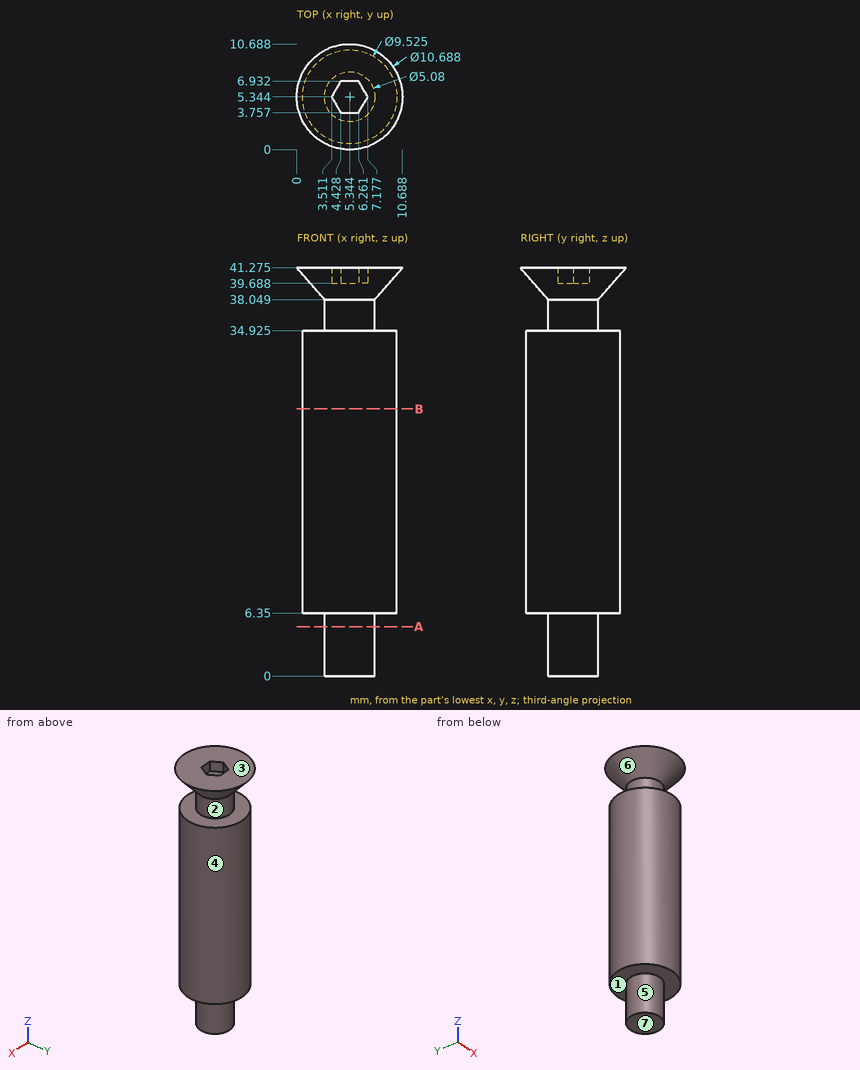
Job drawing, mm, ordinate dimensions from the low corner. One solid piece. A direction names the side the tool comes from. Give positions to 0.01 mm unless a question says otherwise; leave off trailing zeros. Write each loop counter-clockwise with the first axis right and the second up, starting at its lowest first coordinate (ties: lowest second). Pieces come first, ordered by that corner, then holes. Notation, with made-up numbers: (10, 24.5) -> (68, 24.5) arc R5 ccw to (68, 31.5) -> close; hole circle Ø1 at (-23, 39). An arc over 180 degrees is marked (long way). Return JSON: item names as keys, results as strings.
Item 1: Drop flat-ended pins along their axis: pin 1 (1.7 mm diameter, centred on x = 5.5, z = 40, fed in from +Y) (1 decimal); pin 2 (1.5 mm diameter, centred on x = 2, y = 8.5, fed in from -Z); pin 3 (0.8 mm diameter, centred on x = 5, z = 40, fed in from -Y). Give the stop position or say it passes through.
Answer below:
{"pin 1": "stops at y = 10.3", "pin 2": "stops at z = 6.35", "pin 3": "stops at y = 0.77"}
Item 2: Tool access for the marked faces 5, 6 and 7: list every direction of +Z, -Z, +X, -X, +Y, -Y with a clear straight run to the whole face (end or side of a thin tool).
Answer below:
{"face 5": "-Z", "face 6": "none", "face 7": "-Z, +X, -X, +Y, -Y"}
Item 3: Band-saw the part on B-B (z = 27). List the corners of the cut face in (x, y) (1 decimal).
Answer below:
{"outline": "circle Ø9.5 at (5.3, 5.3)"}
Item 4: Two-plate mould, pull along Z, no slides. Class the marked faces 1, 2, 3 and 4: +Z half, -Z half, draft (parallel to the pull), parting line (faces both ways), or undercut.
Answer below:
{"face 1": "-Z half", "face 2": "undercut", "face 3": "+Z half", "face 4": "draft"}
Item 5: Band-saw the part on A-A (z = 5). List the corners of the cut face in (x, y) (1 decimal).
Answer below:
{"outline": "circle Ø5.1 at (5.3, 5.3)"}
Item 6: Drill centre lines: probe 1 along Z at (x, y) = (5.5, 5); probe 2 along Y at (x, z) = (8, 38.5) (1 decimal); probe 3 along Y at (x, z) = (6, 24.5). Where is each one in solid material? Low to high.
Answer below:
{"probe 1": "z = 0 to 39.69", "probe 2": "y = 4.1 to 6.6", "probe 3": "y = 0.63 to 10.06"}
